For this review, take the finished solid that the model builds, in its own axes (mm). A direction names the side the tool comes from. Coordinates: 2 decimals unless noted, no trailing zeros. Loops run counter-clockwise (first coordinate to the right, second up) from the corner with the lowest first, then second, coordinate; pieces in that order, holes last. Notation, with made-up numbers: M 77,45.5 L 84,45.5 A12 cw 84,55.5 Z; hole C -18.75,17 d2. An arc over 180 degrees is marked long. Put each result on its own line as item: value.
```python
from build123d import *

# Parameters (mm, degrees)
SKETCH_1_R      = 1.7500000000000004
SKETCH_1_R_2    = 1.7499999999999998
SKETCH_1_R_3    = 11.25
SKETCH_1_R_4    = 3.2500000000000004
EXTRUDE_1_DEPTH = 4
SKETCH_1_3_R    = 1.7500000000000004
SKETCH_1_3_R_2  = 1.7499999999999998
SKETCH_1_3_R_3  = 11.25
EXTRUDE_2_DEPTH = 7.5
SKETCH_1_4_W    = 8.299999999999999
SKETCH_1_4_H    = 18.999999999999982
EXTRUDE_3_DEPTH = 11
FILLET_1_R      = 2
FILLET_3_R      = 4
SKETCH_1_5_W    = 8.299999999999999
SKETCH_1_5_H    = 12
SKETCH_1_5_R    = 3.2500000000000004
SKETCH_1_5_H_2  = 11.999999999999996
SKETCH_1_5_H_3  = 18.999999999999982
EXTRUDE_4_DEPTH = 5.4
FILLET_2_R      = 1
CHAMFER_1_SIZE  = 0.5


with BuildPart() as part:
    # Эскиз1 → Бобышка-Вытянуть1 (new body)
    with BuildSketch(Plane.XY):
        with BuildLine():
            ThreePointArc((-32.16450146827534, 21.221984437073093), (-35.82965440560809, 19.39826009426678), (-37.30887383412098, 15.581032511990193))
            Line((-37.30887383412098, 15.581032511990193), (-37.30887383412098, -15.418967488009775))
            ThreePointArc((-37.30887383412098, -15.418967488009775), (-35.829654405608096, -19.23619507028637), (-32.16450146827534, -21.059919413092672))
            Line((-32.16450146827534, -21.059919413092672), (20.006045179765074, -25.87421379899061))
            ThreePointArc((20.006045179765074, -25.87421379899061), (27.399020745235244, -22.811943053479965), (30.46129149074589, -15.41896748800979))
            Line((30.46129149074589, -15.418967488009791), (30.461291490745886, 15.581032511990195))
            ThreePointArc((30.461291490745886, 15.581032511990195), (27.39902074523524, 22.97400807746036), (20.006045179765074, 26.036278822971013))
            Line((20.006045179765074, 26.036278822971013), (-32.16450146827534, 21.221984437073093))
        make_face()
        with Locations((-31.643954820235436, -15.418967488009791)):
            Circle(SKETCH_1_R, mode=Mode.SUBTRACT)
        with Locations((-0.643954820235465, -15.418967488009791)):
            Circle(SKETCH_1_R_2, mode=Mode.SUBTRACT)
        with Locations((-16.14395482023548, 0.08103251199020889)):
            Circle(SKETCH_1_R_3, mode=Mode.SUBTRACT)
        with Locations((-31.643954820235436, 15.581032511990195)):
            Circle(SKETCH_1_R, mode=Mode.SUBTRACT)
        with Locations((-0.643954820235465, 15.581032511990195)):
            Circle(SKETCH_1_R, mode=Mode.SUBTRACT)
        with Locations((20.006045179765074, -15.418967488009791)):
            Circle(SKETCH_1_R_4, mode=Mode.SUBTRACT)
        with Locations((20.00604517976507, 15.581032511990195)):
            Circle(SKETCH_1_R_4, mode=Mode.SUBTRACT)
    extrude(amount=EXTRUDE_1_DEPTH)

    # Эскиз1<3> → Бобышка-Вытянуть2 (add)
    with BuildSketch(Plane.XY):
        with BuildLine():
            ThreePointArc((-32.16450146827534, 21.221984437073093), (-35.82965440560809, 19.39826009426678), (-37.30887383412098, 15.581032511990193))
            Line((-37.30887383412098, 15.581032511990193), (-37.30887383412098, -15.418967488009775))
            ThreePointArc((-37.30887383412098, -15.418967488009775), (-35.829654405608096, -19.23619507028637), (-32.16450146827534, -21.059919413092672))
            Line((-32.16450146827533, -21.059919413092675), (5.506045179765067, -24.536154815893063))
            Line((5.506045179765067, -24.536154815893056), (5.506045179765067, 24.698219839873474))
            Line((5.506045179765069, 24.698219839873467), (-32.16450146827534, 21.221984437073093))
        make_face()
        with Locations((-31.643954820235436, -15.418967488009791)):
            Circle(SKETCH_1_3_R, mode=Mode.SUBTRACT)
        with Locations((-0.643954820235465, -15.418967488009791)):
            Circle(SKETCH_1_3_R_2, mode=Mode.SUBTRACT)
        with Locations((-16.14395482023548, 0.08103251199020889)):
            Circle(SKETCH_1_3_R_3, mode=Mode.SUBTRACT)
        with Locations((-31.643954820235436, 15.581032511990195)):
            Circle(SKETCH_1_3_R, mode=Mode.SUBTRACT)
        with Locations((-0.643954820235465, 15.581032511990195)):
            Circle(SKETCH_1_3_R, mode=Mode.SUBTRACT)
    extrude(amount=EXTRUDE_2_DEPTH)

    # Эскиз1<4> → Бобышка-Вытянуть3 (add)
    with BuildSketch(Plane.XY):
        with Locations((20.00604517976507, 0.08103251199020356)):
            Rectangle(SKETCH_1_4_W, SKETCH_1_4_H)
    extrude(amount=EXTRUDE_3_DEPTH)

    # Скругление1
    fillet_1_edges = [part.edges().sort_by_distance(p)[0] for p in [
        (5.506045179765067, -24.53615481589306, 5.75),
        (5.506045179765068, 24.69821983987347, 5.75),
    ]]
    fillet(fillet_1_edges, radius=FILLET_1_R)

    # Скругление3
    # the kernel refuses this fillet: 4 mm, written as the material it adds along each edge
    with BuildSketch(Plane(origin=(3.506045179765067, 22.505162446697916, 4), x_dir=(0.9999802608561372, -0.006283143965559292, 0), z_dir=(0.006283143965559292, 0.9999802608561372, 0))) as fillet_3_piece_1_section:
        with BuildLine():
            CenterArc((5.968626966596891, -4.000000000000001), FILLET_3_R, 90, 82.81924421854171)
            Line((5.968626966596891, 0), (1.9999999999999991, 0))
            Line((1.9999999999999991, 0), (2.0000000000000044, -3.5000000000000018))
        make_face()
    fillet_3_piece_1 = revolve(axis=Axis((3.506045179765067, 22.505162446697916, 4), (0, 0, -1)), revolution_arc=359.64, mode=Mode.PRIVATE)
    fillet_3_piece_1 = split(fillet_3_piece_1, bisect_by=Plane(origin=(3.3222661542347938, 24.49670086454859, 4), z_dir=(0.09188951276513632, -0.9957692089253342, 0)), keep=Keep.TOP, mode=Mode.PRIVATE)
    add(fillet_3_piece_1)
    with BuildSketch(Plane(origin=(5.506045179765067, 22.505162446697916, 4), x_dir=(1.78e-15, 0, 1), z_dir=(0, -1, 0))) as fillet_3_piece_2:
        with BuildLine():
            CenterArc((4.000000000000007, -3.9686269665968847), FILLET_3_R, 97.18075578145837, 82.81924421854171)
            Line((7.05e-15, -3.968626966596892), (0, 0))
            Line((0, 0), (3.500000000000001, 0))
        make_face()
    extrude(amount=44.84825986941543)
    with BuildSketch(Plane(origin=(3.506045179765067, -22.343097422717513, 4), x_dir=(1, 0, 0), z_dir=(0, 1, 0))) as fillet_3_piece_3_section:
        with BuildLine():
            CenterArc((5.968626966596892, -4), FILLET_3_R, 90, 82.81924421854171)
            Line((5.968626966596892, 0), (2, 0))
            Line((2, 0), (2.0000000000000044, -3.500000000000001))
        make_face()
    fillet_3_piece_3 = revolve(axis=Axis((3.506045179765067, -22.343097422717513, 4), (0, 0, -1)), revolution_arc=359.64000000000004, mode=Mode.PRIVATE)
    fillet_3_piece_3 = split(fillet_3_piece_3, bisect_by=Plane(origin=(3.322266154234794, -24.33463584056818, 4), z_dir=(0.09188951276513666, 0.9957692089253342, 0)), keep=Keep.TOP, mode=Mode.PRIVATE)
    add(fillet_3_piece_3)

    # Эскиз1<5> → Бобышка-Вытянуть4 (add)
    # profile 1 of 3: a face of its own
    with BuildSketch(Plane.XY):
        with Locations((20.00604517976507, 15.581032511990195)):
            Rectangle(SKETCH_1_5_W, SKETCH_1_5_H)
        with Locations((20.00604517976507, 15.581032511990195)):
            Circle(SKETCH_1_5_R, mode=Mode.SUBTRACT)
    # profile 2 of 3: a face of its own
    with BuildSketch(Plane.XY):
        with Locations((20.00604517976507, -15.418967488009786)):
            Rectangle(SKETCH_1_5_W, SKETCH_1_5_H_2)
        with Locations((20.006045179765074, -15.418967488009791)):
            Circle(SKETCH_1_5_R, mode=Mode.SUBTRACT)
    # profile 3 of 3: a face of its own
    with BuildSketch(Plane.XY):
        with Locations((20.00604517976507, 0.08103251199020356)):
            Rectangle(SKETCH_1_5_W, SKETCH_1_5_H_3)
    extrude(amount=EXTRUDE_4_DEPTH)

    # Скругление2
    fillet_2_edges = [part.edges().sort_by_distance(p)[0] for p in [
        (15.85604517976507, 21.581032511990195, 4.7),
        (24.15604517976507, -21.418967488009784, 4.7),
        (15.85604517976507, -21.418967488009784, 4.7),
        (24.15604517976507, 21.581032511990195, 4.7),
        (15.85604517976507, -9.418967488009788, 8.2),
        (24.15604517976507, -9.418967488009788, 8.2),
        (24.15604517976507, 9.581032511990195, 8.2),
        (15.85604517976507, 9.581032511990195, 8.2),
    ]]
    fillet(fillet_2_edges, radius=FILLET_2_R)

    # Фаска1
    chamfer_1_edges = [part.edges().sort_by_distance(p)[0] for p in [
        (-27.39395482023548, 0.08103251199021026, 7.5),
    ]]
    chamfer(chamfer_1_edges, length=CHAMFER_1_SIZE)


solid = part.part
```
(1) Add section B-B (z = 2). Write out the cut boundary in (x, y).
Determined:
outline: M -37.31,-15.42 A5.66 ccw -32.16,-21.06 L 20.01,-25.87 A10.46 ccw 30.46,-15.42 L 30.46,15.58 A10.46 ccw 20.01,26.04 L -32.16,21.22 A5.66 ccw -37.31,15.58 Z; hole C -31.64,-15.42 d3.5; hole C -31.64,15.58 d3.5; hole C -16.14,0.08 d22.5; hole C -0.64,-15.42 d3.5; hole C -0.64,15.58 d3.5; hole C 20.01,-15.42 d6.5; hole C 20.01,15.58 d6.5
(2) Add section C-C (x = -0.5). Write out the cut boundary in (y, z), plus the area to 3 significant figures.
Determined:
outline: M -23.98,0 L -17.16,0 L -17.16,7.5 L -23.98,7.5 Z; M -13.67,0 L 13.84,0 L 13.84,7.5 L -13.67,7.5 Z; M 17.33,0 L 24.14,0 L 24.14,7.5 L 17.33,7.5 Z
area: 309 mm^2
(3) For pin 1 (10 mm diameter, centred on x = 8.5, y = 16, fed in from +Z); pin 2 (20 mm diameter, centred on x = -16.14, y = 0.08, fed in from -Z); pin 3 (4 mm diameter, centred on x = -29.5, z = 6.5, fed in from +Y); pin 4 (3 mm diameter, centred on x = 6, z = 8.5, fed in from +Y), all flat-tipped, find the tip position at first contact; note any pin that passes through.
Determined:
pin 1: stops at z = 7.5
pin 2: passes through
pin 3: stops at y = 21.65
pin 4: stops at y = 23.96
(4) Add section A-A (x = 22). Write out the cut boundary in (y, z).
Determined:
outline: M -25.68,0 L -17.99,0 L -17.99,5.4 L -21.42,5.4 L -21.42,4 L -25.68,4 Z; M -12.85,0 L 13.01,0 L 13.01,5.4 L 9.58,5.4 L 9.58,11 L -9.42,11 L -9.42,5.4 L -12.85,5.4 Z; M 18.15,0 L 25.84,0 L 25.84,4 L 21.58,4 L 21.58,5.4 L 18.15,5.4 Z
(5) Tool access review of faces 1 (the flat face through (20, 9.581, 8)), 2 (the cylindrical face through (27.32, -22.89, 1.97)), 3 (the flat face through (24.156, 0, 7)): name each direction out of +Z, -Z, +X, -X, +Y, -Y from which nothing blocks a thin tool from reaching the whole face with its end or side.
Determined:
face 1: +Z, +X, +Y
face 2: +Z, -Z, +X, -Y
face 3: +Z, +X, +Y, -Y
(6) Wall thickness on line 1 along X through (y, z) = (9, 5.5); line 2 along Y through (x, z) = (-32, 1.75); line 3 along X through (y, z) = (-14.5, 6.5): over which ranges is each line inside the solid? List them lowest first. Write a range as [from, to].
Determined:
line 1: x = [-37.31, -23], [-9.29, 6.35], [15.95, 24.06]
line 2: y = [-21.08, -17.13], [-13.71, 13.87], [17.29, 21.24]
line 3: x = [-37.31, -33.13], [-30.15, -2.13], [0.85, 5.77]
(7) Draft analysis for pull direction X (two halves, no side actions). For faces 4 (the cylindrical face through (27.48, 22.89, 1.97)), 5 (the cylindrical face through (-35.79, 19.44, 3.7)), 6 (the cylindrical face through (-25.072, -6.764, 3.451)), state which applies: +X half, -X half, draft (parallel to the pull), parting line (faces both ways), or undercut.
Determined:
face 4: +X half
face 5: -X half
face 6: undercut
